Check sheet for the modelled part. Datum: model origin and axes. Units: mm. A direction names the side the tool comes from. Coordinates: 2 decimals unless noted, no trailing zeros. Loops run counter-clockwise (first coordinate to the right, second up) from the corner with the lowest first, then second, coordinate; pieces in that order, holes last.
```python
from build123d import *

# Parameters (mm, degrees)
F0_W     = 5
F0_H     = 100
F0_W_2   = 50
F0_H_2   = 40
F1_DEPTH = 100
F2_W     = 10
F2_H     = 10
F2_H_2   = 10.6422880292
F3_DEPTH = 20
F4_R     = 10
F5_R     = 10
F6_SIZE  = 5
F7_SIZE  = 5
F8_SIZE2 = 39.99999
F8_SIZE  = 99.99999


# Not quite as in the source:
# - a fillet or chamfer is up to 0.001 mm smaller than in the source, because OpenCascade refuses the exact size


with BuildPart() as f1:
    # F0 (on Right) → F1 (new body)
    with BuildSketch(Plane.YZ):
        with Locations((2.5, 50)):
            Rectangle(F0_W, F0_H)
        Polygon((5, 100), (5, 0), (50, 0), (95, 0), (95, 100), (75, 100), (75, 90), (75, 50), (25, 50), (25, 90), (25, 100), align=None)
        with BuildLine():
            ThreePointArc((57.5, 15), (55.3033008589, 9.6966991411), (50, 7.5))
            ThreePointArc((50, 7.5), (44.6966991411, 20.3033008589), (57.5, 15))
        make_face(mode=Mode.SUBTRACT)
        with Locations((97.5, 50)):
            Rectangle(F0_W, F0_H)
        with Locations((50, 70)):
            Rectangle(F0_W_2, F0_H_2)
    extrude(amount=-F1_DEPTH)

    # F2 (on Front) → F3 (cut)
    with BuildSketch(Plane.XZ):
        with Locations((-80, 15)):
            Rectangle(F2_W, F2_H)
        with Locations((-60, 15)):
            Rectangle(F2_W, F2_H)
        with Locations((-40, 15)):
            Rectangle(F2_W, F2_H)
        with Locations((-20, 15.3211440146)):
            Rectangle(F2_W, F2_H_2)
    extrude(amount=-F3_DEPTH, mode=Mode.SUBTRACT)

    # F4
    f4_edges = [f1.edges().sort_by_distance(p)[0] for p in [
        (-100, 12.5, 100),
    ]]
    fillet(f4_edges, radius=F4_R)

    # F5
    f5_edges = [f1.edges().sort_by_distance(p)[0] for p in [
        (-100, 87.5, 100),
    ]]
    fillet(f5_edges, radius=F5_R)

    # F6
    f6_edges = [f1.edges().sort_by_distance(p)[0] for p in [
        (0, 0, 50),
    ]]
    chamfer(f6_edges, length=F6_SIZE)

    # F7
    f7_edges = [f1.edges().sort_by_distance(p)[0] for p in [
        (0, 100, 50),
    ]]
    chamfer(f7_edges, length=F7_SIZE)

    # F8 (size 100 and 40 in the source; OpenCascade refuses exactly that, so slightly less here)
    f8_edges = [f1.edges().sort_by_distance(p)[0] for p in [
        (0, 50, 90),
    ]]
    f8_side = f1.faces().sort_by_distance((-50, 50, 90))[0]
    chamfer(f8_edges, length=F8_SIZE, length2=F8_SIZE2, reference=f8_side)


with BuildPart() as f1_1:
    # F9: moved
    add(f1.part.moved(Location((100, 0, 0))))


solid = f1_1.part
```
1) Section check D-D on z = 70. Enter the section's corners in (x, y).
Answer sheet:
outline: (0, 0) - (95, 0) - (100, 5) - (100, 25) - (50, 25) - (50, 75) - (100, 75) - (100, 95) - (95, 100) - (0, 100) - close
2) Depth check by flat-ended pin: pin 1 (5 mm diameter, centred on x = 80.5, z = 17, fed in from -Y); pin 2 (1.5 mm diameter, centred on x = 37.5, y = 33.5, fed in from +Z). Enter the tip coordinate at first touch or a pass-through.
Answer sheet:
pin 1: stops at y = 20
pin 2: stops at z = 75.3
3) Mould release check, pull along Y, two halves, no side actions. Record for faces 1 (the flat face through (62, 75, 81)), 2 (the flat face through (15, 10, 15)), 3 (the flat face through (98, 3, 49)): +Y half, -Y half, draft (parallel to the pull), parting line (faces both ways), or undercut.
Answer sheet:
face 1: undercut
face 2: draft
face 3: -Y half
4) Section check A-A on z = 15. Enter the section's corners in (x, y).
Answer sheet:
outline: (0, 0) - (15, 0) - (15, 20) - (25, 20) - (25, 0) - (35, 0) - (35, 20) - (45, 20) - (45, 0) - (55, 0) - (55, 20) - (65, 20) - (65, 0) - (75, 0) - (75, 20) - (85, 20) - (85, 0) - (95, 0) - (100, 5) - (100, 42.5) - (0, 42.5) - close; (0, 57.5) - (100, 57.5) - (100, 95) - (95, 100) - (0, 100) - close
5) Set-up check for faces 4 (the flat face through (60, 10, 10)), 5 (the flat face through (48, 100, 49)), 6 (the flat face through (62, 25, 80)): record each of +Z, -Z, +X, -X, +Y, -Y from which the full face is reachable in a straight line by a thin tool's end or side.
Answer sheet:
face 4: -Y
face 5: +Z, -Z, +X, -X, +Y
face 6: +Z, +X
6) Scan lines: line 1 (Z direction, x = 22.5, y = 6.5); line 2 (Y direction, x = 33, z = 15); line 3 (Z direction, x = 76.5, y = 18). Record each from-to range of solid material in increasing order.
Answer sheet:
line 1: z = 0 to 10, 20 to 100
line 2: y = 0 to 42.5, 57.5 to 100
line 3: z = 0 to 10, 20.64 to 100
7) Section check B-B on x = 78. Enter the section's corners in (y, z), plus the area to 3 significant figures.
Answer sheet:
outline: (0, 0) - (100, 0) - (100, 100) - (75, 100) - (75, 58.8) - (25, 58.8) - (25, 100) - (0, 100) - (0, 20.64) - (20, 20.64) - (20, 10) - (0, 10) - close; hole circle Ø15 at (50, 15)
area: 7,550 mm2
